Part print with two shaded views. Sizes in mm from the minimum x, y, z corner. Coordinates: 2 decimals unless noted, no trailing zeros. Write each loop counter-clockwise with the first axis right and the second up, starting at its lowest first coordinate (ties: lowest second). Pieces come first, ordered by that corner, then holes. Notation, with made-up numbers: M -18,48 L 39,48 A21 cw 39,59 Z; hole C 85.5,62.5 d4. An arc over 180 degrees is marked long. One line per question, with ' | ' between items. Start each with the question number.
(1) Flat gauge pins, fed straight in: pin 1 Ø1 at (x, y) = (2, 9.5) entering from -Z; pin 2 Ø6 at (x, y) = (8, 2.5) entering from -Z. Where does each tip first touch, or does it go through?
(2) Cut at C-C (x = 9.5). Write the cut outline in (y, z), plus the area to 3 significant figures.
(3) Wall check: probe 1 along Z at (x, y) = (4.5, 6); probe 2 along Z at (x, y) = (2, 7); probe 3 along Y at (x, z) = (4.25, 3.75). Give the ranges that are in metal, low to high.
(4) Two-plate mould, pull along Y, no slides. Class the marked faces 1 and 2: +Y half, -Y half, draft (parallel to the pull), parting line (faces both ways), or undercut.
(5) Cut at A-A (y = 6). Write the cut outline in (x, z).
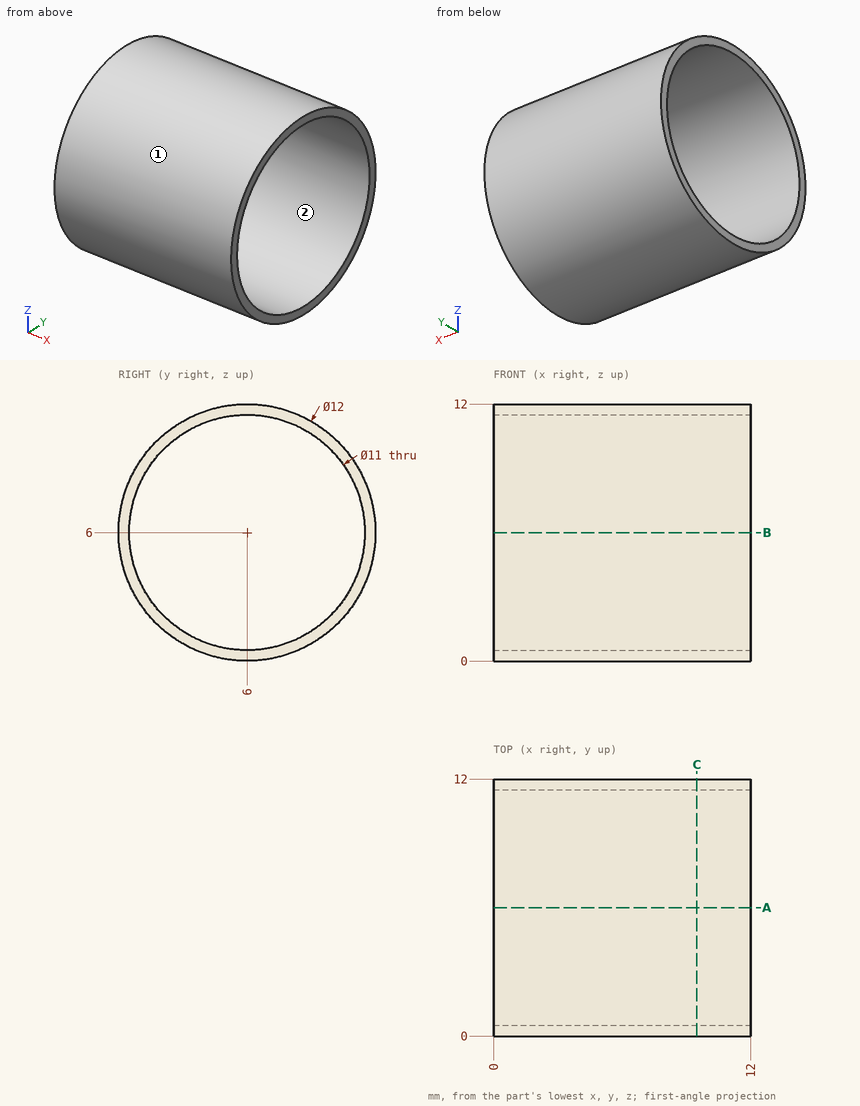
Filled in:
1) pin 1: z = 0.8 | pin 2: z = 0.02
2) outline: C 6,6 d12; hole C 6,6 d11 | area: 18.1 mm²
3) probe 1: 0 to 0.5, 11.5 to 12 | probe 2: 0.08 to 0.59, 11.41 to 11.92 | probe 3: 0.44 to 0.98, 11.02 to 11.56
4) face 1: parting line | face 2: undercut
5) outline: M 0,0 L 12,0 L 12,0.5 L 0,0.5 Z; M 0,11.5 L 12,11.5 L 12,12 L 0,12 Z
